Here's how the part is built. I have some questions about the finished solid (model axes, mm). A direction names the side the tool comes from. Coordinates: 2 decimals unless noted, no trailing zeros. Write each loop counter-clockwise with the first axis right and the second up, starting at its lowest first coordinate (ties: lowest second). Pieces come first, ordered by that corner, then holes.
```python
from build123d import *

# Parameters (mm, degrees)
SKETCH_1_R          = 2.5
EXTRUDE_1_DEPTH     = 4
SKETCH_2_R          = 0.75
CUT_EXTRUDE_1_DEPTH = 10
SKETCH_3_R          = 25.464829655
SKETCH_3_R_2        = 18.5
CUT_EXTRUDE_2_DEPTH = 10


with BuildPart() as part:
    # Эскиз1 → Бобышка-Вытянуть1 (new body)
    with BuildSketch(Plane(origin=(0, 0, 0), x_dir=(0, 0, -1), z_dir=(1, 0, 0))):
        with BuildLine():
            Line((7.85991422, -1.49055335), (13.754849795, -2.608468346))
            ThreePointArc((13.754849795, -2.608468346), (13.231778891, 9.584616389), (5.051373997, 18.641431188))
            ThreePointArc((5.051373997, 18.641431188), (-18.822494325, 4.328168593), (-3.59851409, -18.975511385))
            Line((-3.59851409, -18.975511385), (-1.490553351, -7.859914224))
            ThreePointArc((-1.490553351, -7.859914224), (1.865542593, -2.738688528), (7.85991422, -1.49055335))
        make_face()
        Circle(SKETCH_1_R, mode=Mode.SUBTRACT)
    extrude(amount=EXTRUDE_1_DEPTH)

    # Эскиз2 → Вырез-Вытянуть1 (cut)
    with BuildSketch(Plane(origin=(4, 0, 0), x_dir=(0, 0, -1), z_dir=(1, 0, 0))):
        with Locations((-11.107644425, -9.32042034)):
            Circle(SKETCH_2_R)
        with Locations((11.107644425, 9.32042034)):
            Circle(SKETCH_2_R)
    extrude(amount=-CUT_EXTRUDE_1_DEPTH, mode=Mode.SUBTRACT)

    # Эскиз3 → Вырез-Вытянуть2 (cut)
    with BuildSketch(Plane(origin=(4, 0, 0), x_dir=(0, 0, -1), z_dir=(1, 0, 0))):
        Circle(SKETCH_3_R)
        Circle(SKETCH_3_R_2, mode=Mode.SUBTRACT)
    extrude(amount=-CUT_EXTRUDE_2_DEPTH, mode=Mode.SUBTRACT)


solid = part.part
```
1) Will these pins go through, and if not, where does the flat tip stop? pin 1 (1.5 mm diameter, centred on x = 1, y = -2.5, fed in from -Z); pin 2 (1.5 mm diameter, centred on x = 2.5, z = -8, fed in from +Y); pin 3 (1 mm diameter, centred on x = 3.5, y = -1, fed in from -Z).
Values follow:
pin 1: stops at z = -14
pin 2: stops at y = 17.02
pin 3: stops at z = -14.28
2) Imagine slicing it at B-B on y = 0. Please give me the cut outline in (x, z), then the cut area to 3 significant figures.
Values follow:
outline: (0, -14.36) - (4, -14.36) - (4, -2.5) - (0, -2.5) - close; (0, 2.5) - (4, 2.5) - (4, 18.5) - (0, 18.5) - close
area: 111 mm2
3) Imagine slicing it at C-C on x = 2.9. Please give me the cut outline in (y, z).
Values follow:
outline: (-18.18, 3.45) - (-7.86, 1.49) arc R8 cw to (-1.49, -7.86) - (-2.61, -13.75) arc R18 ccw to (16.69, -7.97) arc R18.5 ccw (long way) to start; hole circle Ø1.5 at (-9.32, 11.11); hole circle Ø5 at (0, 0); hole circle Ø1.5 at (9.32, -11.11)
4) We'd pull the mould along Y, two halves only. Please class faces 3 (the face through (2.028, -8.814, 11.66)), 4 (the face through (4, 4, 2)), 5 (the face through (1.97, -2.79, -1.79)), 6 (the face through (2.03, 6.17, 17.44)): pulls with the +Y half, pulls with the -Y half, needs draft (parallel to the pull), parting line crosses it, or undercut.
Values follow:
face 3: undercut
face 4: needs draft
face 5: pulls with the -Y half
face 6: parting line crosses it
5) Imagine slicing it at D-D on z = -4.5. Please give me the cut outline in (x, y), then the cut area to 3 significant figures.
Values follow:
outline: (0, -1.57) - (4, -1.57) - (4, 17.94) - (0, 17.94) - close
area: 78.1 mm2
6) On a 3-axis mill with a long thin cutter (end or side, diameter ignored), from which of +Z, -Z, +X, -X, +Y, -Y can I reach the whole of each face in a straight line? I mean faces 1 (the face through (1.972, -2.042, -10.766)), 2 (the face through (0, 4, 2)). Say none if no direction works.
Values follow:
face 1: +X, -X, -Y
face 2: +Z, -Z, -X, +Y, -Y
7) I need wall thicknesses on probe 1 along Z at (x, y) = (1.8, 0.5); probe 2 along Z at (x, y) = (3.2, 1); probe 3 along Y at (x, z) = (3.85, -10.5). Which ranges of each line are inside material? Lowest first, please.
Values follow:
probe 1: z = -14.43 to -2.45, 2.45 to 18.49
probe 2: z = -14.49 to -2.29, 2.29 to 18.47
probe 3: y = -1.99 to 8.88, 9.76 to 14.17
8) Imagine slicing it at A-A on z = 0. Please give me the cut outline in (x, y).
Values follow:
outline: (0, -4.51) - (4, -4.51) - (4, -2.5) - (0, -2.5) - close; (0, 2.5) - (4, 2.5) - (4, 18.5) - (0, 18.5) - close
